Input: part model. Units: mm. Frame: model coordinates. Face numbers are marked on the shaded views. A direction names the side the tool comes from. Give positions to 0.01 mm unless a question says otherwise; leave off trailing zeros. Order: outer loops, then holes, each group sorted by start corner. A loop starts at its lowest first (then second) coordinate and runs counter-clockwise, first axis right, second up. Notation, with made-up numbers: (58.25, -39) - (112.25, -39) arc R15 cw to (112.25, -28) - close; hole circle Ø1 at (41.5, -38). An arc over 180 degrees is marked (long way). Answer in a Markdown table with one row per item. Add a question column.
1. Section query A-A on x = -5. Return loops of the section in (y, z).
2. Mould query, pull axis Y, two halves, no side actions, for the marked faces 4, 5 and 6. Classes: released by +Y, released by -Y, zero draft, split by the parting line, or undercut.
3. Section query B-B on z = 7.5. Return loops of the section in (x, y), and give its area (3 significant figures).
4. Access query for the marked faces 1, 2 and 3. Directions: +Z, -Z, +X, -X, +Y, -Y. A direction counts if a zero-diameter tool reaches every point of the face in a straight line with its end or side. Return the directions, or none.
5. Ray query, line 1 (X direction, y = -12.75, z = 12); line 2 (Y direction, x = 5, z = 31.75); line 3 (X direction, y = -17, z = 12). Return the intervals inside material, ascending. Write a range as [from, to].
6. Section query C-C on x = -29.5. Return loops of the section in (y, z).
7. Section query D-D on y = -20.5. Return loops of the section in (x, z), and give its area (3 significant figures).
8. Contact query for flat-ended pins moving along their axis: pin 1 (3 mm diameter, centred on x = 27, y = -10, fed in from -Z); pin 2 (2 mm diameter, centred on x = -1, y = -22.5, fed in from +Z); pin 3 (12 mm diameter, centred on y = -4.5, z = 8.5, fed in from +X); pin 4 (8 mm diameter, centred on x = -6, y = -7.5, fed in from -Z). Output: stop coordinate, or through.
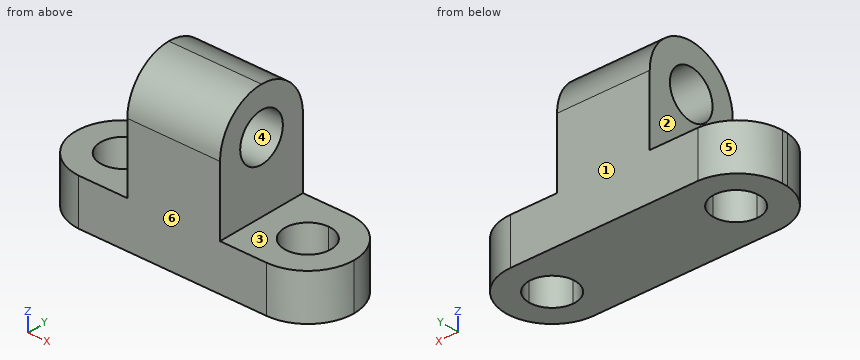
```python
from build123d import *

# Parameters (mm, degrees)
F1_DEPTH = 25.4
F3_DEPTH = 50.801
F5_DEPTH = 12.701
F7_DEPTH = 12.701
F9_DEPTH = 12.701


with BuildPart() as f1:
    # F0 (on Front) → F1 (new body)
    with BuildSketch(Plane.XZ):
        Polygon((-38.1542058029, 12.7), (-38.1542058029, 0), (38.0457941971, 0), (38.0457941971, 12.7), (12.6457941971, 12.7), (12.6457941971, 44.45), (-12.7542058029, 44.45), (-12.7542058029, 12.7), align=None)
    extrude(amount=F1_DEPTH)

    # F2 (on face) → F3 (cut, through all)
    with BuildSketch(Plane.YZ.offset(12.6457941971)):
        with BuildLine():
            Line((-19.2294398129, 31.75), (-6.1705601871, 31.75))
            ThreePointArc((-6.1705601871, 31.75), (-12.7, 38.2794398129), (-19.2294398129, 31.75))
        make_face()
        with BuildLine():
            ThreePointArc((-19.2294398129, 31.75), (-12.7, 25.2205601871), (-6.1705601871, 31.75))
            Line((-6.1705601871, 31.75), (-19.2294398129, 31.75))
        make_face()
        with BuildLine():
            ThreePointArc((-25.4, 31.75), (-21.6802561211, 40.7302561211), (-12.7, 44.45))
            Line((-12.7, 44.45), (-25.4, 44.45))
            Line((-25.4, 44.45), (-25.4, 31.75))
        make_face()
        with BuildLine():
            ThreePointArc((-12.7, 44.45), (-3.7197438789, 40.7302561211), (0, 31.75))
            Line((0, 31.75), (0, 44.45))
            Line((0, 44.45), (-12.7, 44.45))
        make_face()
    extrude(amount=-F3_DEPTH, mode=Mode.SUBTRACT)

    # F4 (on face) → F5 (cut, through all)
    with BuildSketch(Plane.XY.offset(12.7)):
        with BuildLine():
            Line((-25.1679819405, -25.2168271691), (-25.9211060628, -25.2168271691))
            ThreePointArc((-25.9211060628, -25.2168271691), (-25.5445440017, -25.2224491047), (-25.1679819405, -25.2168271691))
        make_face()
        with BuildLine():
            ThreePointArc((25.3457941971, -6.3600277162), (19.0058219133, -12.7), (25.3457941971, -19.0399722838))
            Line((25.3457941971, -19.0399722838), (25.3457941971, -6.3600277162))
        make_face()
        with BuildLine():
            Line((25.3457941971, -6.3600277162), (25.3457941971, -19.0399722838))
            ThreePointArc((25.3457941971, -19.0399722838), (29.8288315915, -17.1830373944), (31.6857664808, -12.7))
            ThreePointArc((31.6857664808, -12.7), (29.8288315915, -8.2169626056), (25.3457941971, -6.3600277162))
        make_face()
        with BuildLine():
            Line((-25.1679819405, -18.9560678934), (-25.1679819405, -6.2607592757))
            ThreePointArc((-25.1679819405, -6.2607592757), (-31.5156362493, -12.6084135845), (-25.1679819405, -18.9560678934))
        make_face()
        with BuildLine():
            ThreePointArc((-18.8203276317, -12.6084135845), (-20.6795125341, -8.1199441781), (-25.1679819405, -6.2607592757))
            Line((-25.1679819405, -6.2607592757), (-25.1679819405, -18.9560678934))
            ThreePointArc((-25.1679819405, -18.9560678934), (-20.6795125341, -17.0968829909), (-18.8203276317, -12.6084135845))
        make_face()
        with BuildLine():
            ThreePointArc((25.3457941971, 0), (34.3260503181, -3.7197438789), (38.0457941971, -12.7))
            Line((38.0457941971, -12.7), (38.0457941971, 0))
            Line((38.0457941971, 0), (25.3457941971, 0))
        make_face()
        with BuildLine():
            ThreePointArc((38.0457941971, -12.7), (34.3260503181, -21.6802561211), (25.3457941971, -25.4))
            Line((25.3457941971, -25.4), (38.0457941971, -25.4))
            Line((38.0457941971, -25.4), (38.0457941971, -12.7))
        make_face()
    extrude(amount=-F5_DEPTH, mode=Mode.SUBTRACT)

    # F6 (on face) → F7 (cut, through all)
    with BuildSketch(Plane.XY.offset(12.7)):
        with BuildLine():
            ThreePointArc((-38.1542058029, -12.2175221546), (-34.4600291378, -3.683299298), (-25.9211060628, 0))
            Line((-25.9211060628, 0), (-38.1542058029, 0))
            Line((-38.1542058029, 0), (-38.1542058029, -12.2175221546))
        make_face()
    extrude(amount=-F7_DEPTH, mode=Mode.SUBTRACT)

    # F8 (on face) → F9 (cut, through all)
    with BuildSketch(Plane.XY.offset(12.7)):
        with BuildLine():
            Line((-38.1542058029, -25.4), (-26.090927422, -25.4))
            ThreePointArc((-26.090927422, -25.4), (-34.2975944615, -21.8697418221), (-38.1542058029, -13.8112893863))
            Line((-38.1542058029, -13.8112893863), (-38.1542058029, -25.4))
        make_face()
    extrude(amount=-F9_DEPTH, mode=Mode.SUBTRACT)


solid = f1.part
```
Answer:
| question | item | result |
|---|---|---|
| 1 | outline | (-25.4, 0) - (0, 0) - (0, 31.75) arc R12.7 ccw to (-25.4, 31.75) - close; hole circle Ø13.06 at (-12.7, 31.75) |
| 2 | face 4 | undercut |
| 2 | face 5 | released by +Y |
| 2 | face 6 | released by -Y |
| 3 | outline | (-38.15, -13.81) arc R12.71 ccw to (-26.09, -25.4) - (25.35, -25.4) arc R12.7 ccw to (25.35, 0) - (-25.92, 0) arc R12.61 ccw to (-38.15, -12.22) - close; hole circle Ø12.7 at (-25.17, -12.61); hole (-25.92, -25.22) arc R12.61 ccw to (-25.17, -25.22) - close; hole circle Ø12.68 at (25.35, -12.7) |
| 3 | area | 1,550 mm² |
| 4 | face 1 | +Z, -Z, +X, -X, +Y |
| 4 | face 2 | +Z, -X, +Y, -Y |
| 4 | face 3 | +Z, +X, +Y, -Y |
| 5 | line 1 | x = [-38.15, -31.51], [-18.82, 19.01], [31.69, 38.05] |
| 5 | line 2 | y = [-25.4, -19.23], [-6.17, 0] |
| 5 | line 3 | x = [-37.45, -29.75], [-20.58, 20.69], [30, 37.3] |
| 6 | outline | (-24.77, 0) - (-17.25, 0) - (-17.25, 12.7) - (-24.77, 12.7) - close; (-7.97, 0) - (-0.63, 0) - (-0.63, 12.7) - (-7.97, 12.7) - close |
| 7 | outline | (-35.53, 0) - (35.37, 0) - (35.37, 12.7) - (12.65, 12.7) - (12.65, 41.77) - (-12.75, 41.77) - (-12.75, 12.7) - (-35.53, 12.7) - close |
| 7 | area | 1,640 mm² |
| 8 | pin 1 | passes through |
| 8 | pin 2 | stops at z = 40.91 |
| 8 | pin 3 | stops at x = 37.85 |
| 8 | pin 4 | stops at z = 0 |
